Could you check a few things on this drawing? It's one solid part, dimensions in mm from its lowest x, y, z. A direction names the side the tool comes from. Give positions to 0.01 mm unless a question says otherwise; leave off trailing zeros. Loops run counter-clockwise (first coordinate to the right, second up) from the corner with the lowest first, then second, coordinate; pieces in that order, holes last. Notation, with made-up numbers: (-23, 81.25) -> (22, 81.25) arc R32 ccw to (22, 110.25) -> close; hole circle Ø10 at (57, 37.25). An arc over 180 degrees is marked (long way). Use CSV: the item, a comma, the result in double quotes.
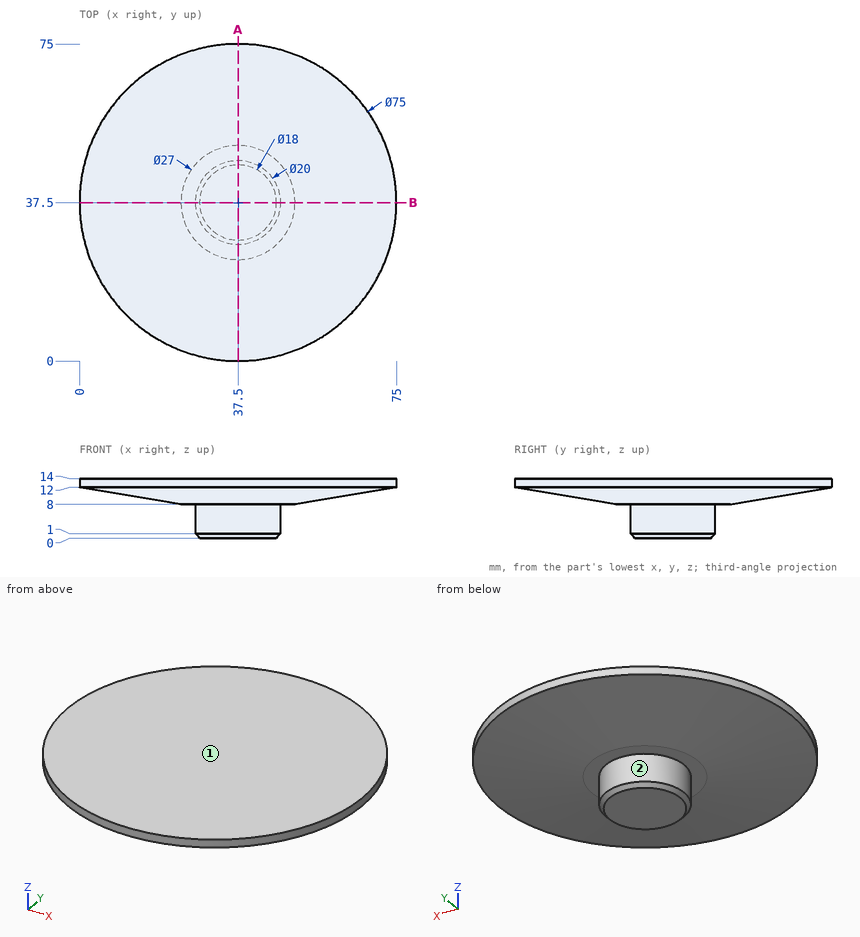
(1) Will these pins go through, and if not, where does the flat tip stop? pin 1 Ø1 at (x, z) = (43, 12) entering from -Y; pin 2 Ø2 at (x, z) = (50, 11.5) entering from +Y; pin 3 Ø2 at (y, z) = (49.5, 12.5) entering from +X.
Answer sheet:
pin 1,"stops at y = 0.33"
pin 2,"stops at y = 73.15"
pin 3,"stops at x = 73.35"
(2) If I drill on L1, parallel to Z at x = 47, y = 32; L2, parallel to Y at x = 38, z = 3.5; L3, parallel to X at y = 36.5, z = 13.25, over which ranges is the centre line in solid material (lowest first)? Write a range as from..to.
Answer sheet:
L1,"z = 8..14"
L2,"y = 27.51..47.49"
L3,"x = 0.01..74.99"
(3) If we section it at A-A, the plane x = 37.5: Write out the boundary of the cut face in (y, z), then the cut area to 3 significant figures.
Answer sheet:
outline,"(0, 12) -> (24, 8) -> (27.5, 8) -> (27.5, 1) -> (28.5, 0) -> (46.5, 0) -> (47.5, 1) -> (47.5, 8) -> (51, 8) -> (75, 12) -> (75, 14) -> (0, 14) -> close"
area,"513 mm2"
(4) Which directions (+Z, -Z, +X, -X, +Y, -Y) give clear straight access to the entire face, cutting with the end or side of a thin tool? Please do the marked faces 1 and 2.
Answer sheet:
face 1,"+Z, +X, -X, +Y, -Y"
face 2,"-Z"
